Source: CAD feature listing. Evaluate the final solid. Frame: model axes, mm. Face numbers are marked on the shaded views. A direction names the side the tool comes from. Give positions to 0.01 mm unless a question says otherwise; leave off trailing zeros. Loops run counter-clockwise (first coordinate to the right, second up) from the corner with the lowest first, then second, coordinate; pieces in that order, holes last. Notation, with made-up numbers: (51.5, -14) -> (98.5, -14) arc R18 cw to (98.5, 10) -> close; hole circle Ø5 at (23, -14.75). An arc over 180 degrees is marked (long way). Answer as a JSON object with one key per item and string values. Group by question number.
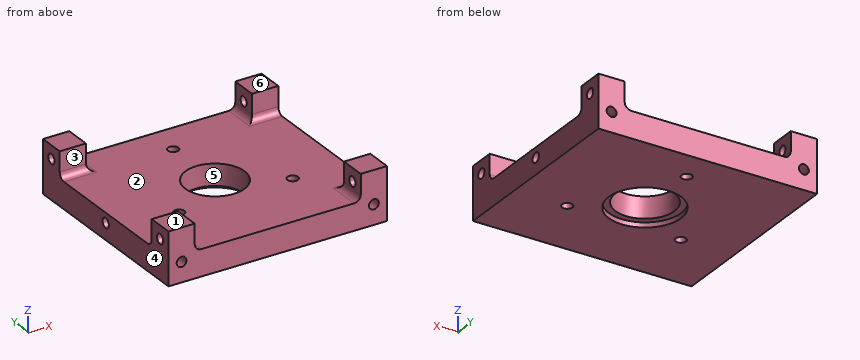
from build123d import *

# Parameters (mm, degrees)
SKETCH_1_W          = 66.6
SKETCH_1_H          = 60
SKETCH_1_R          = 1.6
SKETCH_1_R_2        = 9
EXTRUDE_1_DEPTH     = 8
SKETCH_3_W          = 8
SKETCH_3_H          = 8
EXTRUDE_2_DEPTH     = 8
SKETCH_4_R          = 1.5
CUT_EXTRUDE_1_DEPTH = 8
CUT_EXTRUDE_START   = -8
SKETCH_5_R          = 1.5
CUT_EXTRUDE_2_DEPTH = 8
SKETCH_6_R          = 1.5
CUT_EXTRUDE_3_DEPTH = 8
SKETCH_7_R          = 1.5
CUT_EXTRUDE_4_DEPTH = 8
FILLET_1_R          = 2
SKETCH_8_R          = 11
CUT_EXTRUDE_5_DEPTH = 1.5


with BuildPart() as part:
    # 草图1 → 凸台-拉伸1 (new body)
    with BuildSketch(Plane.XY):
        Rectangle(SKETCH_1_W, SKETCH_1_H)
        with Locations((0, 20)):
            Circle(SKETCH_1_R, mode=Mode.SUBTRACT)
        with Locations((17.320508076, -10)):
            Circle(SKETCH_1_R, mode=Mode.SUBTRACT)
        with Locations((-17.320508076, -10)):
            Circle(SKETCH_1_R, mode=Mode.SUBTRACT)
        Circle(SKETCH_1_R_2, mode=Mode.SUBTRACT)
    extrude(amount=EXTRUDE_1_DEPTH)

    # 草图3 → 凸台-拉伸2 (add)
    with BuildSketch(Plane.XY.offset(8)):
        with Locations((-29.3, 26)):
            Rectangle(SKETCH_3_W, SKETCH_3_H)
        with Locations((-29.3, -26)):
            Rectangle(SKETCH_3_W, SKETCH_3_H)
        with Locations((29.3, -26)):
            Rectangle(SKETCH_3_W, SKETCH_3_H)
        with Locations((29.3, 26)):
            Rectangle(SKETCH_3_W, SKETCH_3_H)
    extrude(amount=EXTRUDE_2_DEPTH)

    # 草图4 → 切除-拉伸1 (cut)
    with BuildSketch(Plane.ZY.offset(33.3)):
        with Locations((12, 26)):
            Circle(SKETCH_4_R)
        with Locations(Location((12, -26, 0), (0, 0, 180))):
            Circle(SKETCH_4_R)
        with Locations((5, 0)):
            Circle(SKETCH_4_R)
    extrude(amount=-CUT_EXTRUDE_1_DEPTH, mode=Mode.SUBTRACT)

    # 草图5 → 切除-拉伸2 (cut)
    with BuildSketch(Plane(origin=(33.3, 0, 0), x_dir=(0, 0, -1), z_dir=(1, 0, 0)).offset(CUT_EXTRUDE_START)):
        with Locations((-12, -26)):
            Circle(SKETCH_5_R)
        with Locations(Location((-12, 26, 0), (0, 0, 180))):
            Circle(SKETCH_5_R)
        with Locations(Location((-5, 0, 0), (0, 0, 180))):
            Circle(SKETCH_5_R)
    extrude(amount=CUT_EXTRUDE_2_DEPTH, mode=Mode.SUBTRACT)

    # 草图6 → 切除-拉伸3 (cut)
    with BuildSketch(Plane(origin=(0, 30, 0), x_dir=(1, 0, 0), z_dir=(0, 1, 0))):
        with Locations(Location((-29.3, -6, 0), (0, 0, 180))):
            Circle(SKETCH_6_R)
        with Locations((29.3, -6)):
            Circle(SKETCH_6_R)
    extrude(amount=-CUT_EXTRUDE_3_DEPTH, mode=Mode.SUBTRACT)

    # 草图7 → 切除-拉伸4 (cut)
    with BuildSketch(Plane.XZ.offset(30).offset(CUT_EXTRUDE_START)):
        with Locations((29.3, 6)):
            Circle(SKETCH_7_R)
        with Locations(Location((-29.3, 6, 0), (0, 0, 180))):
            Circle(SKETCH_7_R)
    extrude(amount=CUT_EXTRUDE_4_DEPTH, mode=Mode.SUBTRACT)

    # 圆角1
    fillet_1_edges = [part.edges().sort_by_distance(p)[0] for p in [
        (-29.3, 22, 8),
        (-25.3, 26, 8),
        (-25.3, -26, 8),
        (-29.3, -22, 8),
        (29.3, -22, 8),
        (25.3, -26, 8),
        (25.3, 26, 8),
        (29.3, 22, 8),
    ]]
    fillet(fillet_1_edges, radius=FILLET_1_R)

    # 草图8 → 切除-拉伸5 (cut)
    with BuildSketch(Plane(origin=(0, 0, 0), x_dir=(-1, 0, 0), z_dir=(0, 0, -1))):
        Circle(SKETCH_8_R)
    extrude(amount=-CUT_EXTRUDE_5_DEPTH, mode=Mode.SUBTRACT)


solid = part.part
(1) Section query D-D on y = 0. Return the cut outline in (x, z).
(2) Mould query, pull axis X, two halves, no side actions, for the marked faces 4, 5 and 6. Classes: pulls with the +X half, pulls with the -X half, needs draft (parallel to the pull), parting line crosses it, or undercut.
(3) Material intervals for line 1 (Y direction, x = -27, z = 12); line 2 (Y direction, x = -30, z = 5); line 3 (Z direction, x = 29, y = 26), sorted ascending. Write a range as from..to.
(4) Access query for the marked faces 1, 2 and 3. Directions: +Z, -Z, +X, -X, +Y, -Y. A direction counts if a zero-diameter tool reaches every point of the face in a straight line with its end or side. Return the directions, or none.
(5) Section query C-C on x = 0. Return the cut outline in (y, z), plus the area to 3 significant figures.
(6) Section query B-B on z = 12. State how many separate pieces and enclosed holes the cut face has, plus the area to 3 significant figures.
(7) First-contact query: pin 1 (2 mm diameter, centred on x = 26.5, y = 1, fed in from +Z); pin 2 (17.5 mm diameter, centred on x = 0, y = 0, fed in from +Z); pin 3 (2.5 mm diameter, centred on x = -29.3, z = 6, fed in from +Y); pin 4 (0.9 mm diameter, centred on x = 28.5, z = 6, fed in from -Y). Flat tips, straight axial feed; report the tip coordinate or a pass-through.
(8) Section query A-A on y = -26. Return the cut outline in (x, z), plus the area to 3 significant figures.
Result:
{
 "1": {"outline": "(-33.3, 0) -> (-11, 0) -> (-11, 1.5) -> (-9, 1.5) -> (-9, 8) -> (-33.3, 8) -> (-33.3, 6.5) -> (-25.3, 6.5) -> (-25.3, 3.5) -> (-33.3, 3.5) -> close; (9, 1.5) -> (11, 1.5) -> (11, 0) -> (33.3, 0) -> (33.3, 3.5) -> (25.3, 3.5) -> (25.3, 6.5) -> (33.3, 6.5) -> (33.3, 8) -> (9, 8) -> close"},
 "2": {"face 4": "pulls with the -X half", "face 5": "undercut", "face 6": "needs draft"},
 "3": {"line 1": "-30..-27.5, -24.5..-22, 22..24.5, 27.5..30", "line 2": "-22..-1.5, 1.5..22", "line 3": "0..4.53, 7.47..10.5, 13.5..16"},
 "4": {"face 1": "+Z, +X, -X, +Y, -Y", "face 2": "+Z", "face 3": "+Z, +X, -X"},
 "5": {"outline": "(-30, 0) -> (-11, 0) -> (-11, 1.5) -> (-9, 1.5) -> (-9, 8) -> (-30, 8) -> close; (9, 1.5) -> (11, 1.5) -> (11, 0) -> (18.4, 0) -> (18.4, 8) -> (9, 8) -> close; (21.6, 0) -> (30, 0) -> (30, 8) -> (21.6, 8) -> close", "area": "304 mm²"},
 "6": {"separate pieces": "8", "enclosed holes": "0", "area": "160 mm²"},
 "7": {"pin 1": "z = 8", "pin 2": "through", "pin 3": "y = 22", "pin 4": "y = -22"},
 "8": {"outline": "(-33.3, 0) -> (33.3, 0) -> (33.3, 10.5) -> (25.3, 10.5) -> (25.3, 10) arc R2 cw to (23.3, 8) -> (-23.3, 8) arc R2 cw to (-25.3, 10) -> (-25.3, 10.5) -> (-33.3, 10.5) -> close; (-33.3, 13.5) -> (-25.3, 13.5) -> (-25.3, 16) -> (-33.3, 16) -> close; (25.3, 13.5) -> (33.3, 13.5) -> (33.3, 16) -> (25.3, 16) -> close; hole circle Ø3 at (-29.3, 6); hole circle Ø3 at (29.3, 6)", "area": "600 mm²"}
}
